```python
from build123d import *

# Parameters (mm, degrees)
ESQUISSE1_W          = 59
ESQUISSE1_H          = 23
BOSS_EXTRU_4_DEPTH   = 10
ESQUISSE1_H_2        = 41
BOSS_EXTRU_4_2_DEPTH = 10
ESQUISSE1_H_3        = 6
BOSS_EXTRU_4_3_DEPTH = 10
ESQUISSE1_6_W        = 59
ESQUISSE1_6_H        = 70
ESQUISSE1_6_H_2      = 10
BOSS_EXTRU_5_DEPTH   = 9


with BuildPart() as part:
    # Esquisse1 → Boss.-Extru.4 (new body)
    with BuildSketch(Plane.XY):
        with Locations((-16.034238867, -28.643003421)):
            Rectangle(ESQUISSE1_W, ESQUISSE1_H)
    extrude(amount=BOSS_EXTRU_4_DEPTH)



with BuildPart() as body_2:
    # Esquisse1 → Boss.-Extru.4 2 (new body)
    with BuildSketch(Plane.XY):
        with Locations((-16.034238867, -70.643003421)):
            Rectangle(ESQUISSE1_W, ESQUISSE1_H_2)
    extrude(amount=BOSS_EXTRU_4_2_DEPTH)


with BuildPart() as body_3:
    # Esquisse1 → Boss.-Extru.4 3 (new body)
    with BuildSketch(Plane.XY):
        with Locations((-16.034238867, -104.143003421)):
            Rectangle(ESQUISSE1_W, ESQUISSE1_H_3)
    extrude(amount=BOSS_EXTRU_4_3_DEPTH)


with BuildPart() as part_1:
    add(part.part)

    add(body_2.part)  # Boss.-Extru.5 merges body 2

    add(body_3.part)  # Boss.-Extru.5 merges body 3
    # Esquisse1_6 → Boss.-Extru.5 (add)
    with BuildSketch(Plane.XY):
        with Locations((-16.034238867, 17.856996579)):
            Rectangle(ESQUISSE1_6_W, ESQUISSE1_6_H)
        with Locations((-16.034238867, -45.143003421)):
            Rectangle(ESQUISSE1_6_W, ESQUISSE1_6_H_2)
        with Locations((-16.034238867, -96.143003421)):
            Rectangle(ESQUISSE1_6_W, ESQUISSE1_6_H_2)
    extrude(amount=BOSS_EXTRU_5_DEPTH)


solid = part_1.part
```
Verification items for the finished model (mm, model axes). A direction names the side the tool comes from. Coordinates: 2 decimals unless noted, no trailing zeros. Loops run counter-clockwise (first coordinate to the right, second up) from the corner with the lowest first, then second, coordinate; pieces in that order, holes last. Notation, with made-up numbers: (-5.5, 38.5) - (19.5, 38.5) arc R35 cw to (19.5, 76.5) - close; hole circle Ø10 at (43, 54.25). An arc over 180 degrees is marked (long way). Answer as a JSON object with one key per item and string values.
(1) Go/stop test with flat-tipped pins: pin 1 Ø3 at (x, y) = (-14.5, 4) entering from +Z; pin 2 Ø1.1 at (x, z) = (-26.5, 9.5) entering from +Y; pin 3 Ø0.5 at (x, z) = (-14, 9.5) entering from +Y. Record where each tip stops, or that it passes through.
Response:
{"pin 1": "stops at z = 9", "pin 2": "stops at y = 52.86", "pin 3": "stops at y = -17.14"}
(2) Mould release check, pull along Y, two halves, no side actions. Record for faces 4 (the flat face through (-16, -26, 0)), 5 (the flat face through (-16, -96, 9)), 6 (the flat face through (-16, -107.143, 5)), 7 (the flat face through (-16, 52.857, 4)): pulls with the +Y half, pulls with the -Y half, needs draft (parallel to the pull), parting line crosses it, or undercut.
Response:
{"face 4": "needs draft", "face 5": "undercut", "face 6": "pulls with the -Y half", "face 7": "pulls with the +Y half"}
(3) Cross-section at B-B, the plane y = -12. Record the boundary of the cut face in (x, z).
Response:
{"outline": "(-45.53, 0) - (13.47, 0) - (13.47, 9) - (-45.53, 9) - close"}
(4) Cross-section at A-A, the plane x = 8. Record the boundary of the cut face in (y, z).
Response:
{"outline": "(-107.14, 0) - (52.86, 0) - (52.86, 9) - (-17.14, 9) - (-17.14, 10) - (-40.14, 10) - (-40.14, 9) - (-50.14, 9) - (-50.14, 10) - (-91.14, 10) - (-91.14, 9) - (-101.14, 9) - (-101.14, 10) - (-107.14, 10) - close"}
(5) Access from +Z, -Z, +X, -X, +Y, -Y to the whole of each face (thin tool, end or side, straight path). Record for faces 1 (the flat face through (-16, 18, 9)), 2 (the flat face through (-16, -45, 9)), 3 (the flat face through (-45.534, -28, 5)).
Response:
{"face 1": "+Z, +X, -X, +Y", "face 2": "+Z, +X, -X", "face 3": "+Z, -Z, -X, +Y, -Y"}
(6) Scan line: line 1 along Z through (x, y) = (-41, -6). Record every from-to range of solid material in increasing order.
Response:
{"line 1": "z = 0 to 9"}
